Input: part model. Units: mm. Frame: model coordinates. Face numbers are marked on the shaded views. A direction names the side the tool comes from. Round coordinates to 2 decimals unless told otherwise and drop trailing zeros. Order: outer loops, then holes, each group sorted by start corner. A loop starts at its lowest first (then second) coordinate and runs counter-clockwise, first axis right, second up.
Item 1: Cut plane A-A on z = 10. Output: boundary loops of the cut face in (x, y).
Item 2: Cut plane B-B on x = -5. Output: boundary loops of the cut face in (y, z).
Item 3: Line query: L1, parallel to X at y = 2.5, z = -13; L2, parallel to X at y = 2.1, z = 16; L3, parallel to Z at x = 4.5, y = 0.55. Output: solid intervals per line, ascending.
Item 4: Mould query, pull axis Z, two halves, no side actions, for the marked faces 1, 2, 3 and 4. Classes: released by +Z, released by -Z, zero draft, split by the parting line, or undercut.
Item 5: Cut plane C-C on y = 2. Output: boundary loops of the cut face in (x, z), then the cut area to 3 significant figures.
Item 6: Reachability of the marked faces 5 and 6 from +Z, -Z, +X, -X, +Y, -Y: full face, straight path, thin tool, end or side. Return the list, or none.
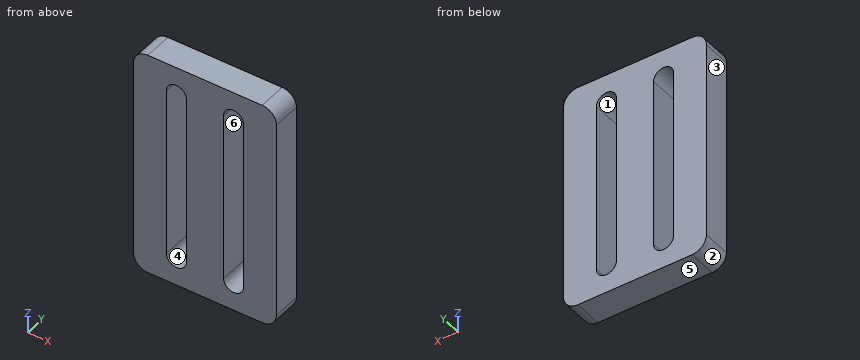
```python
from build123d import *

# Parameters (mm, degrees)
SKETCH1_W           = 25
SKETCH1_H           = 40
BOSS_EXTRUDE1_DEPTH = 5
CUT_EXTRUDE1_DEPTH  = 5
FILLET1_R           = 2.5


with BuildPart() as part:
    # Sketch1 → Boss-Extrude1 (new body)
    with BuildSketch(Plane(origin=(0, 0, 0), x_dir=(1, 0, 0), z_dir=(0, 1, 0))):
        Rectangle(SKETCH1_W, SKETCH1_H)
    extrude(amount=BOSS_EXTRUDE1_DEPTH)

    # Sketch2 → Cut-Extrude1 (cut)
    with BuildSketch(Plane(origin=(0, 5, 0), x_dir=(1, 0, 0), z_dir=(0, 1, 0))):
        with BuildLine():
            Line((-3.25, 15), (-3.25, -15))
            ThreePointArc((-3.25, -15), (-5, -16.75), (-6.75, -15))
            Line((-6.75, -15), (-6.75, 15))
            ThreePointArc((-6.75, 15), (-5, 16.75), (-3.25, 15))
        make_face()
        with BuildLine():
            Line((3.25, 15), (3.25, -15))
            ThreePointArc((3.25, -15), (5, -16.75), (6.75, -15))
            Line((6.75, -15), (6.75, 15))
            ThreePointArc((6.75, 15), (5, 16.75), (3.25, 15))
        make_face()
    extrude(amount=-CUT_EXTRUDE1_DEPTH, mode=Mode.SUBTRACT)

    # Fillet1
    fillet1_edges = [part.edges().sort_by_distance(p)[0] for p in [
        (12.5, 2.5, 20),
        (-12.5, 2.5, 20),
        (-12.5, 2.5, -20),
        (12.5, 2.5, -20),
    ]]
    fillet(fillet1_edges, radius=FILLET1_R)


solid = part.part
```
From the geometry:
1. outline: (-12.5, 0) - (-6.75, 0) - (-6.75, 5) - (-12.5, 5) - close; (-3.25, 0) - (3.25, 0) - (3.25, 5) - (-3.25, 5) - close; (6.75, 0) - (12.5, 0) - (12.5, 5) - (6.75, 5) - close
2. outline: (0, -20) - (5, -20) - (5, -16.75) - (0, -16.75) - close; (0, 16.75) - (5, 16.75) - (5, 20) - (0, 20) - close
3. L1: x = -12.5 to -6.75, -3.25 to 3.25, 6.75 to 12.5
3. L2: x = -12.5 to -6.44, -3.56 to 3.56, 6.44 to 12.5
3. L3: z = -20 to -16.68, 16.68 to 20
4. face 1: undercut
4. face 2: released by -Z
4. face 3: zero draft
4. face 4: undercut
5. outline: (-12.5, -17.5) arc R2.5 ccw to (-10, -20) - (10, -20) arc R2.5 ccw to (12.5, -17.5) - (12.5, 17.5) arc R2.5 ccw to (10, 20) - (-10, 20) arc R2.5 ccw to (-12.5, 17.5) - close; hole (-6.75, -15) arc R1.75 ccw to (-3.25, -15) - (-3.25, 15) arc R1.75 ccw to (-6.75, 15) - close; hole (3.25, -15) arc R1.75 ccw to (6.75, -15) - (6.75, 15) arc R1.75 ccw to (3.25, 15) - close
5. area: 765 mm2
6. face 5: -Z, +X, -X, +Y, -Y
6. face 6: +Y, -Y
